Part model, mm, in its own coordinate system. A direction names the side the tool comes from. Give positions to 0.01 mm unless a question says otherwise; leave off trailing zeros. Write each loop counter-clockwise with the first axis right and the second up, starting at its lowest first coordinate (ties: lowest second). Pieces come first, ordered by that corner, then holes.
from build123d import *

# Parameters (mm, degrees)
SKETCH1_W              = 203.2
SKETCH1_H              = 152.4
BASE_DEPTH             = 5.334
CENTER_CUT_DEPTH       = 255.056000827
CENTER_CUT_DEPTH_BACK  = 255.056000827
SKETCH4_W              = 5.334
SKETCH4_H              = 19.05
SKETCH4_H_2            = 57.15
SLOTS_DEPTH            = 255.056000827
LEADING_EDGE_FILLET_R  = 25.4
WEIGHT_REDUCTION_DEPTH = 255.056000827


with BuildPart() as part:
    # Sketch1 → Base (new body)
    with BuildSketch(Plane(origin=(0, 0, 0), x_dir=(1, 0, 0), z_dir=(0, 1, 0))):
        with Locations((101.6, 76.2)):
            Rectangle(SKETCH1_W, SKETCH1_H)
    extrude(amount=BASE_DEPTH)

    # Sketch2 → Center Cut (cut, two sides: drawn at the far end of the back side and taken through both)
    with BuildSketch(Plane(origin=(0, 5.334, 0), x_dir=(1, 0, 0), z_dir=(0, 1, 0)).offset(-CENTER_CUT_DEPTH_BACK)):
        Polygon((-127.880204408, 592.259835398), (32.215682926, 152.4), (63.5, 66.447045256), (101.6, 44.45), (139.7, 66.447045256), (170.984317074, 152.4), (331.080204408, 592.259835398), (331.080204408, 1528.437955069), (-127.880204408, 1528.437955069), align=None)
    extrude(amount=CENTER_CUT_DEPTH + CENTER_CUT_DEPTH_BACK, mode=Mode.SUBTRACT)

    # Sketch4 → Slots (cut, through all)
    with BuildSketch(Plane(origin=(0, 5.334, 0), x_dir=(1, 0, 0), z_dir=(0, 1, 0))):
        with Locations((2.667, 104.775)):
            Rectangle(SKETCH4_W, SKETCH4_H)
        with Locations((200.533, 28.575)):
            Rectangle(SKETCH4_W, SKETCH4_H_2)
        with Locations((2.667, 28.575)):
            Rectangle(SKETCH4_W, SKETCH4_H_2)
        with Locations((200.533, 104.775)):
            Rectangle(SKETCH4_W, SKETCH4_H)
    extrude(amount=-SLOTS_DEPTH, mode=Mode.SUBTRACT)

    # Leading Edge Fillet
    leading_edge_fillet_edges = [part.edges().sort_by_distance(p)[0] for p in [
        (170.984317074, 2.667, -152.4),
        (32.215682926, 2.667, -152.4),
    ]]
    fillet(leading_edge_fillet_edges, radius=LEADING_EDGE_FILLET_R)

    # Sketch5 → Weight Reduction (cut, through all)
    with BuildSketch(Plane(origin=(0, 5.334, 0), x_dir=(1, 0, 0), z_dir=(0, 1, 0))):
        Polygon((14.430411455, 12.7), (188.769588545, 12.7), (188.769588545, 63.027385411), (101.6, 25.4), (14.430411455, 63.027385411), align=None)
        with BuildLine():
            Line((14.430411455, 139.7), (14.430411455, 79.156722924))
            Line((14.430411455, 79.156722924), (51.123931231, 63.31769886))
            Line((51.123931231, 63.31769886), (26.364507739, 131.34365582))
            ThreePointArc((26.364507739, 131.34365582), (21.714832197, 137.403230962), (14.430411455, 139.7))
        make_face()
        with BuildLine():
            Line((176.835492261, 131.34365582), (152.076068769, 63.31769886))
            Line((152.076068769, 63.31769886), (188.769588545, 79.156722924))
            Line((188.769588545, 79.156722924), (188.769588545, 139.7))
            ThreePointArc((188.769588545, 139.7), (181.485167803, 137.403230962), (176.835492261, 131.34365582))
        make_face()
    extrude(amount=-WEIGHT_REDUCTION_DEPTH, mode=Mode.SUBTRACT)


solid = part.part
1) 3-axis set-ups, long thin cutter, end or side, ignore diameter. For faces 4 (the flat face through (3, 3, -57.15)), 5 (the flat face through (3, 3, -95.25)), 6 (the flat face through (170.17, 2.7, -71.13)): which of +Z, -Z, +X, -X, +Y, -Y reach the whole face in a straight line?
Check result:
face 4: +Z, -X, +Y, -Y
face 5: -X, +Y, -Y
face 6: +Y, -Y
2) Saw through at B-B (z = -125). Write the cut outline in (x, y).
Check result:
outline: (0, 0) - (14.43, 0) - (14.43, 5.33) - (0, 5.33) - close; (28.67, 0) - (42.19, 0) - (42.19, 5.33) - (28.67, 5.33) - close; (161.01, 0) - (174.53, 0) - (174.53, 5.33) - (161.01, 5.33) - close; (188.77, 0) - (203.2, 0) - (203.2, 5.33) - (188.77, 5.33) - close
3) Saw through at A-A (x = 99). Write the cut outline in (y, z), and give its area (3 significant figures).
Check result:
outline: (0, -45.95) - (5.33, -45.95) - (5.33, -26.52) - (0, -26.52) - close; (0, -12.7) - (5.33, -12.7) - (5.33, 0) - (0, 0) - close
area: 171 mm2
4) Flat gauge pins, fed straight in: P1, Ø1, axis at y = 4.5, z = -54, coming from the -X side; P2, Ø2.5, axis at y = 2.5, z = -106, coming from the +X side; P3, Ø2.5, axis at x = 201.5, y = 2.5, coming from the +Z side. Where does each tip first touch, or does it go through?
Check result:
P1: stops at x = 5.33
P2: stops at x = 197.87
P3: stops at z = -57.15
5) Saw through at D-D (z = -29). Write the cut outline in (x, y).
Check result:
outline: (5.33, 0) - (14.43, 0) - (14.43, 5.33) - (5.33, 5.33) - close; (93.26, 0) - (109.94, 0) - (109.94, 5.33) - (93.26, 5.33) - close; (188.77, 0) - (197.87, 0) - (197.87, 5.33) - (188.77, 5.33) - close
6) Drill centre lines: L1, parallel to X at y = 0.2, z = -79; L2, parallel to X at y = 4.35, z = -50.5; L3, parallel to Z at x = 183, y = 5.15. Where is each one in solid material? Low to high.
Check result:
L1: x = 0 to 14.79, 45.42 to 58.93, 144.27 to 157.78, 188.41 to 203.2
L2: x = 5.33 to 14.43, 43.45 to 91.12, 112.08 to 159.75, 188.77 to 197.87
L3: z = -151.74 to -138.31, -76.67 to -60.54, -12.7 to 0
7) Mould opens along X. For faces 1 (the flat face through (100, 5.334, -43)), 2 (the cylindrical face through (21.804, 2.704, -137.341)), 3 (the flat face through (5.334, 3, -105)) say: +X half, -X half, draft (parallel to the pull), parting line (faces both ways), or undercut.
Check result:
face 1: draft
face 2: undercut
face 3: -X half
8) Saw through at C-C (x = 44.5). Write the cut outline in (y, z).
Check result:
outline: (0, -118.65) - (5.33, -118.65) - (5.33, -81.52) - (0, -81.52) - close; (0, -66.18) - (5.33, -66.18) - (5.33, -50.05) - (0, -50.05) - close; (0, -12.7) - (5.33, -12.7) - (5.33, 0) - (0, 0) - close
